The listing builds one solid part. Answer for the finished solid, in the listing's coordinates (mm). Face numbers are marked on the shaded views. Coordinates: 2 decimals unless noted, no trailing zeros. Order: outer loops, then holes, each group sorted by start corner. A loop starts at its lowest first (then second) coordinate and runs counter-clockwise, first axis right, second up. Notation, with made-up numbers: (58, 73.25) -> (72, 73.25) arc R27 ccw to (72, 93.25) -> close; hole circle Ø6 at (58.25, -26). An arc over 180 degrees is marked (long way). Return JSON: item names as keys, results as strings.
```python
from build123d import *

# Parameters (mm, degrees)
SKETCH1_W           = 30.5
SKETCH1_H           = 85
BOSS_EXTRUDE1_DEPTH = 2
CUT_EXTRUDE1_DEPTH  = 2
SKETCH5_W           = 0.8
SKETCH5_H           = 4
BOSS_EXTRUDE2_DEPTH = 3
SKETCH6_R           = 1
CUT_EXTRUDE2_DEPTH  = 0.8
FILLET1_R           = 2
FILLET2_R           = 2
SKETCH7_W           = 30.5
SKETCH7_H           = 2
BOSS_EXTRUDE3_DEPTH = 16
SKETCH8_W           = 30.5
SKETCH8_H           = 80
BOSS_EXTRUDE4_DEPTH = 1.8
SKETCH9_W           = 28.5
SKETCH9_H           = 80
CUT_EXTRUDE3_DEPTH  = 1.8
SKETCH10_W          = 28.9
SKETCH10_H          = 2
CUT_EXTRUDE4_DEPTH  = 1
SKETCH11_W          = 9
SKETCH11_H          = 6
CUT_EXTRUDE5_DEPTH  = 2


with BuildPart() as part:
    # Sketch1 → Boss-Extrude1 (new body)
    with BuildSketch(Plane(origin=(0, 0, 0), x_dir=(1, 0, 0), z_dir=(0, 1, 0))):
        Rectangle(SKETCH1_W, SKETCH1_H)
    extrude(amount=BOSS_EXTRUDE1_DEPTH)

    # Sketch2 → Cut-Extrude1 (cut)
    with BuildSketch(Plane(origin=(0, 2, 0), x_dir=(1, 0, 0), z_dir=(0, 1, 0))):
        Polygon((14.45, 42.5), (-14.45, 42.5), (-14.45, 24.5), (-14.45, 22.5), (14.45, 22.5), (14.45, 24.5), align=None)
    extrude(amount=-CUT_EXTRUDE1_DEPTH, mode=Mode.SUBTRACT)

    # Sketch5 → Boss-Extrude2 (add)
    with BuildSketch(Plane(origin=(0, 2, 0), x_dir=(1, 0, 0), z_dir=(0, 1, 0))):
        with Locations((-14.85, 40.5)):
            Rectangle(SKETCH5_W, SKETCH5_H)
    boss_extrude2 = extrude(amount=BOSS_EXTRUDE2_DEPTH)

    # Sketch6 → Cut-Extrude2 (cut)
    with BuildSketch(Plane.ZY.offset(15.25)):
        with Locations((-40.5, 2)):
            Circle(SKETCH6_R)
    cut_extrude2 = extrude(amount=-CUT_EXTRUDE2_DEPTH, mode=Mode.SUBTRACT)

    # Mirror1: Boss-Extrude2, Cut-Extrude2 across plane
    add(boss_extrude2.mirror(Plane(origin=(0, 0, 0), x_dir=(0, 0, 1), z_dir=(1, 0, 0))))
    add(cut_extrude2.mirror(Plane(origin=(0, 0, 0), x_dir=(0, 0, 1), z_dir=(1, 0, 0))), mode=Mode.SUBTRACT)

    # Fillet1
    fillet1_edges = [part.edges().sort_by_distance(p)[0] for p in [
        (-14.85, 0, -42.5),
        (-14.85, 5, -42.5),
        (-14.85, 5, -38.5),
    ]]
    fillet(fillet1_edges, radius=FILLET1_R - 0.0001)  # a hair under: the kernel refuses the full size

    # Fillet2
    fillet2_edges = [part.edges().sort_by_distance(p)[0] for p in [
        (14.85, 0, -42.5),
        (14.85, 5, -38.5),
        (14.85, 5, -42.5),
    ]]
    fillet(fillet2_edges, radius=FILLET2_R - 0.0001)  # a hair under: the kernel refuses the full size

    # Sketch7 → Boss-Extrude3 (add)
    with BuildSketch(Plane.XY.offset(42.5)):
        with Locations((0, 1)):
            Rectangle(SKETCH7_W, SKETCH7_H)
    extrude(amount=BOSS_EXTRUDE3_DEPTH)

    # Sketch8 → Boss-Extrude4 (add)
    with BuildSketch(Plane(origin=(0, 2, 0), x_dir=(1, 0, 0), z_dir=(0, 1, 0))):
        with Locations((0, -18.5)):
            Rectangle(SKETCH8_W, SKETCH8_H)
    extrude(amount=BOSS_EXTRUDE4_DEPTH)

    # Sketch9 → Cut-Extrude3 (cut)
    with BuildSketch(Plane(origin=(0, 3.8, 0), x_dir=(1, 0, 0), z_dir=(0, 1, 0))):
        with Locations((0, -18.5)):
            Rectangle(SKETCH9_W, SKETCH9_H)
    extrude(amount=-CUT_EXTRUDE3_DEPTH, mode=Mode.SUBTRACT)

    # Sketch10 → Cut-Extrude4 (cut)
    with BuildSketch(Plane(origin=(0, 0, -22.5), x_dir=(-1, 0, 0), z_dir=(0, 0, -1))):
        with Locations((0, 1)):
            Rectangle(SKETCH10_W, SKETCH10_H)
    extrude(amount=-CUT_EXTRUDE4_DEPTH, mode=Mode.SUBTRACT)

    # Sketch11 → Cut-Extrude5 (cut)
    with BuildSketch(Plane(origin=(0, 2, 0), x_dir=(1, 0, 0), z_dir=(0, 1, 0))):
        with Locations((-9.75, -50.5)):
            Rectangle(SKETCH11_W, SKETCH11_H)
    extrude(amount=-CUT_EXTRUDE5_DEPTH, mode=Mode.SUBTRACT)


solid = part.part
```
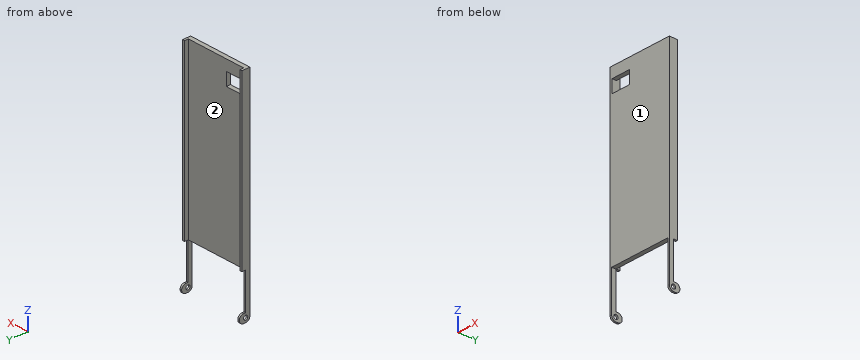
Item 1: Flat-ended cylindrical pins translate along their axes: pin 1 (0.8 mm diameter, centred on x = 14.5, z = 21, fed in from +Y); pin 2 (1.2 mm diameter, centred on y = 2, z = -40.5, fed in from -X); pin 3 (1.5 mm diameter, centred on x = 0, y = 1.5, fed in from -Z); pin 4 (6 mm diameter, centred on x = 1, z = 10, fed in from +Y). Find the tip coordinate at first contact, or state that the pin passes through.
Answer list:
{"pin 1": "y = 3.8", "pin 2": "through", "pin 3": "z = -21.5", "pin 4": "y = 2"}
Item 2: The part is cut by section C-C on z = 39. Determine the outline of the cut face in (x, y), plus the area to 3 significant figures.
Answer list:
{"outline": "(-15.25, 0) -> (15.25, 0) -> (15.25, 3.8) -> (14.25, 3.8) -> (14.25, 2) -> (-14.25, 2) -> (-14.25, 3.8) -> (-15.25, 3.8) -> close", "area": "64.6 mm2"}
Item 3: The part is cut by section B-B on z = -36. Determine the outline of the cut face in (x, y).
Answer list:
{"outline": "(-15.25, 0) -> (-14.45, 0) -> (-14.45, 2) -> (-15.25, 2) -> close; (14.45, 0) -> (15.25, 0) -> (15.25, 2) -> (14.45, 2) -> close"}
Item 4: The part is cut by section A-A on x = -10. Determine the outline of the cut face in (y, z).
Answer list:
{"outline": "(0, -21.5) -> (2, -21.5) -> (2, 47.5) -> (0, 47.5) -> close; (0, 53.5) -> (2, 53.5) -> (2, 58.5) -> (0, 58.5) -> close"}
Item 5: The part is cut by section D-D on x = 3. Determine the outline of the cut face in (y, z), plus the area to 3 significant figures.
Answer list:
{"outline": "(0, -21.5) -> (2, -21.5) -> (2, 58.5) -> (0, 58.5) -> close", "area": "160 mm2"}
Item 6: Determine the mould class of the marked faces 1 and 2 for opening direction X: pulls with the +X half, pulls with the -X half, needs draft (parallel to the pull), parting line crosses it, or undercut.
Answer list:
{"face 1": "needs draft", "face 2": "undercut"}
Item 7: Find the intervals of material crossed by probe 1 along X at (y, z) = (3.4, 44.5); probe 2 along X at (y, z) = (0.95, -22); probe 3 along Z at (x, y) = (-6, 0.5), in increasing order.
Answer list:
{"probe 1": "-15.25 to -14.25, 14.25 to 15.25", "probe 2": "-15.25 to -14.45, 14.45 to 15.25", "probe 3": "-21.5 to 47.5, 53.5 to 58.5"}
